The figure shows three views and two pictorial views of one solid part (mm, origin at its lowest corner). Answer the questions. A direction names the side the tool comes from. Coordinates: 2 decimals unless noted, no trailing zeros. Order: outer loops, then holes, each group sorted by start corner. A loop starts at its lowest first (then second) coordinate and runs counter-clockwise, first axis right, second up. Notation, with made-up numbers: M 58.25,47 L 88.25,47 A20 ccw 88.25,72 Z; hole C -5,-11 d11. An arc over 180 degrees is marked long. Write item = value, one per line. Start each with the question number.
Q1. Find section C-C on z = 10. Give the vertices of the cut face in (x, y), and give its area (3 significant figures).
Q2. A tool of negligible diameter and unlimited length cuts with its end or side. For the marked faces 4 and 5, from which of +Z, -Z, +X, -X, +Y, -Y can it reach the whole face along a straight path? Write none if from no direction.
Q3. Find section B-B on y = 26.25. Give the vertices of the cut face in (x, z).
Q4. Each of these flat-tipped pins is pushed along its axis until it touches: P1, Ø3, axis at x = 26.75, y = 8.75, coming from the +Z side; P2, Ø2, axis at x = 18, y = 13, coming from the -Z side; P3, Ø4, axis at x = 8.25, y = 8.75, coming from the +Z side. Where does it stop, or does it pass through?
Q5. Straight lines are drawn through the part: line 1 along X through (y, z) = (26.25, 3); line 2 along Y through (x, z) = (8.25, 8.5); line 3 along Y through (x, z) = (26, 3.25) (1 decimal). For each, find the intervals that lie inside material, in ascending order.
Q6. Find section D-D on y = 17.5. Give the vertices of the cut face in (x, z).
Q7. Find section A-A on x = 26.75. Give the vertices of the cut face in (y, z), and give its area (3 significant figures).
Q8. Determine the mould class of the marked faces 1, 2 and 3 for opening direction Y: released by +Y, released by -Y, zero draft, split by the parting line, or undercut.
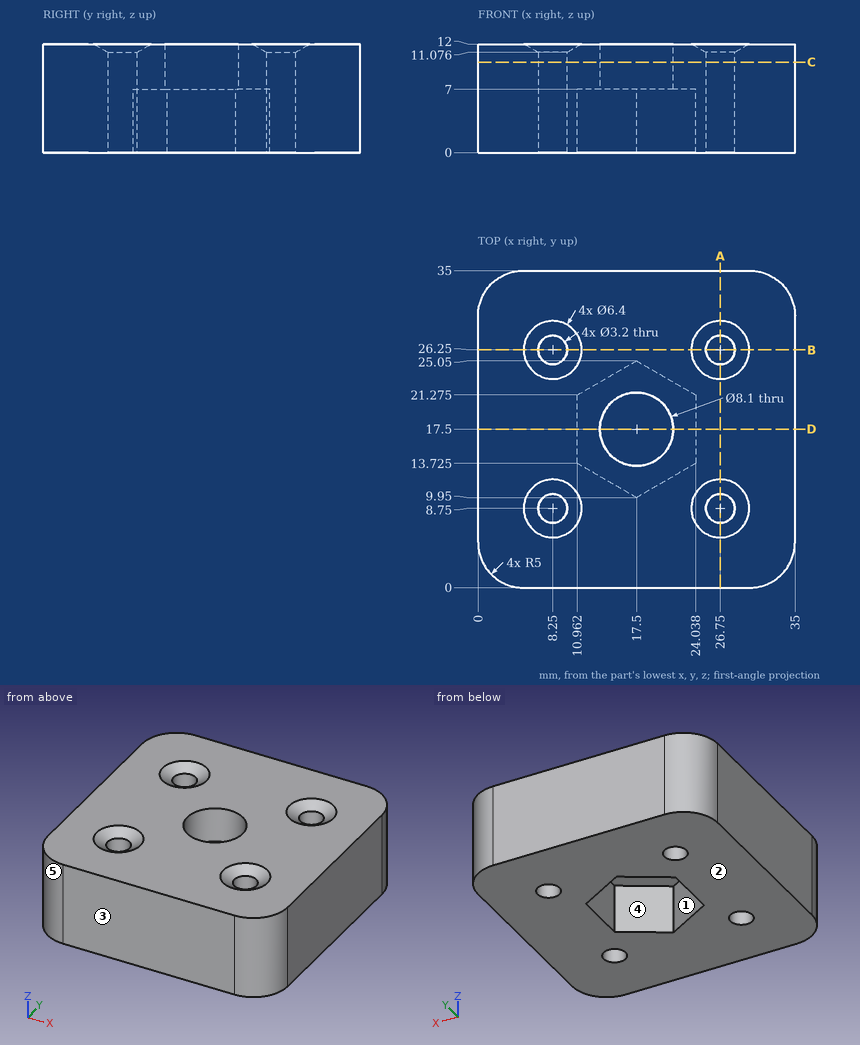
Findings below:
q1.outline = M 0,5 A5 ccw 5,0 L 30,0 A5 ccw 35,5 L 35,30 A5 ccw 30,35 L 5,35 A5 ccw 0,30 Z; hole C 8.25,8.75 d3.2; hole C 8.25,26.25 d3.2; hole C 17.5,17.5 d8.1; hole C 26.75,8.75 d3.2; hole C 26.75,26.25 d3.2
q1.area = 1,120 mm^2
q2.face_4 = -Z
q2.face_5 = +Z, -Z, -X, -Y
q3.outline = M 0,0 L 6.65,0 L 6.65,11.08 L 5.05,12 L 0,12 Z; M 9.85,0 L 25.15,0 L 25.15,11.08 L 23.55,12 L 11.45,12 L 9.85,11.08 Z; M 28.35,0 L 35,0 L 35,12 L 29.95,12 L 28.35,11.08 Z
q4.P1 = through
q4.P2 = 7
q4.P3 = 11.31
q5.line_1 = 0 to 6.65, 9.85 to 25.15, 28.35 to 35
q5.line_2 = 0 to 7.15, 10.35 to 24.65, 27.85 to 35
q5.line_3 = 0 to 7.3, 10.2 to 24.8, 27.7 to 35
q6.outline = M 0,0 L 10.96,0 L 10.96,7 L 13.45,7 L 13.45,12 L 0,12 Z; M 21.55,7 L 24.04,7 L 24.04,0 L 35,0 L 35,12 L 21.55,12 Z
q7.outline = M 0,0 L 7.15,0 L 7.15,11.08 L 5.55,12 L 0,12 Z; M 10.35,0 L 24.65,0 L 24.65,11.08 L 23.05,12 L 11.95,12 L 10.35,11.08 Z; M 27.85,0 L 35,0 L 35,12 L 29.45,12 L 27.85,11.08 Z
q7.area = 340 mm^2
q8.face_1 = undercut
q8.face_2 = zero draft
q8.face_3 = released by -Y
